Design review of the part built by this model. Coordinates are the model's own, in mm. A direction names the side the tool comes from. Give positions to 0.01 mm unless a question says otherwise; leave off trailing zeros. Write each loop counter-clockwise with the first axis right and the second up, starting at its lowest first coordinate (ties: lowest second). Pieces come first, ordered by that corner, then holes. Notation, with made-up numbers: (66.25, 55.25) -> (113.25, 55.25) arc R27 ccw to (113.25, 91.25) -> close; hole circle Ø6 at (-7.75, -39.75). An arc over 180 degrees is marked (long way). Put each result on its own line as item: value. Start each with the question number.
Autodesk Inventor part; units mm, degrees
ref_plane "YZ Plane" through (0, 0, 0) normal (1, 0, 0) x (0, 1, 0)
ref_plane "XZ Plane" through (0, 0, 0) normal (0, 1, 0) x (-1, 0, 0)
ref_plane "XY Plane" through (0, 0, 0) normal (0, 0, 1) x (1, 0, 0)
sketch "Sketch1" plane through (0, 0, 0) normal (0, 1, 0) x (-1, 0, 0)
  line L0 (11.1125, 9.525) -> (-11.1125, 9.525)
  line L1 (-11.1125, 9.525) -> (-11.1125, -9.525)
  line L2 (-11.1125, -9.525) -> (11.1125, -9.525)
  line L3 (11.1125, -9.525) -> (11.1125, 9.525)
  line L4 (11.1125, 9.525) -> (-11.1125, -9.525) construction
  line L5 (-11.1125, 9.525) -> (11.1125, -9.525) construction
  point P0 (0, 0)
  dimension "d0" = 22.225
  dimension "d1" = 19.05
extrude "Plate1" add sketch "Sketch1" along normal blind 1.524
sketch "Sketch2" plane through (-11.1125, 0, -8.001) normal (0, 0, -1) x (-1, 0, 0)
  line L0 (-22.225, 0) -> (0, 0)
  line L1 (0, 0) -> (0, 15.875)
  line L2 (0, 15.875) -> (-22.225, 15.875)
  line L3 (-22.225, 15.875) -> (-22.225, 0)
edge flange "Flange1" height 15.875 angle 90 thickness 1.524 bend radius 1.524 thickness toward (0, 0, -1) relief tear relief width 1.524 relief depth 0.762 edges at (0, 1.524, -9.525) wall of the first edge with corners at (11.1125, 0, -8.001) (-11.1125, 0, -8.001) (-11.1125, 15.875, -8.001) (11.1125, 15.875, -8.001)
bend "Bend1"
corner "Corner1"
sketch "Sketch3" plane through (0, 1.524, 0) normal (0, 1, 0) x (1, 0, 0)
  line L0 (11.1125, 6.477) -> (-11.1125, 6.477)
  line L1 (-11.1125, -9.525) -> (-11.1125, 6.477)
  line L2 (11.1125, -9.525) -> (-11.1125, -9.525)
  line L3 (11.1125, 6.477) -> (11.1125, -9.525)
  line L4 (-11.1125, -1.524) -> (11.1125, -1.524) construction
  line L5 (0, 6.477) -> (0, -9.525) construction
  circle A0 centre (0, -1.524) radius 2.2479
  line L6 (-5.1562, -1.524) -> (5.1562, -1.524) construction
  line L7 (-5.1562, 0.7239) -> (5.1562, 0.7239)
  line L8 (5.1562, -3.7719) -> (-5.1562, -3.7719)
  arc A1 (-5.1562, 0.7239) -> (-5.1562, -3.7719) centre (-5.1562, -1.524) ccw
  arc A2 (5.1562, -3.7719) -> (5.1562, 0.7239) centre (5.1562, -1.524) ccw
  point P0 (0, 0)
  dimension "d13" = 16.002
  dimension "d14" = 22.225
  dimension "d24" = 4.4958
  dimension "d25" = 3.7084
sketch "Sketch4" plane through (-11.1125, 15.875, -8.001) normal (0, 0, 1) x (1, 0, 0)
  line L0 (0, -12.827) -> (22.225, -12.827)
  line L1 (22.225, 0) -> (22.225, -12.827)
  line L2 (22.225, 0) -> (0, 0)
  line L3 (0, 0) -> (0, -12.827)
  line L4 (0, -6.4135) -> (22.225, -6.4135) construction
  line L5 (22.225, 0) -> (22.225, -12.827) construction
  line L6 (11.1125, -12.827) -> (11.1125, 0) construction
  line L7 (22.225, 0) -> (0, 0) construction
  point P0 (11.1125, -15.875)
  point P1 (11.1125, -6.4135)
  dimension "d15" = 22.225
  dimension "d16" = 12.827
hole "Hole1" at (0, 9.4615, -8.001) direction (0, 0, -1) diameter 4.4958 depth 1.524 tip angle 118
extrude "Cut1" cut sketch "Sketch3" against normal blind 1.524 contours A0 | A0 L7 A2 L8 | A0 L8 A1 L7
sketch "Sketch7" plane through (11.1125, 15.875, -9.525) normal (0, 0, -1) x (-1, 0, 0)
  line L0 (0, 0) -> (22.225, 0)
  line L1 (22.225, -15.875) -> (0, -15.875)
  line L2 (0, -12.827) -> (22.225, -12.827)
  point P0 (11.1125, -15.875)
  dimension "d28" = 15.875
  dimension "d29" = 12.827
  dimension "d30" = 22.225
sketch "Sketch8" plane through (0, 0, 0) normal (0, -1, 0) x (1, 0, 0)
  arc A0 (-5.1562, 3.7719) -> (-5.1562, -0.7239) centre (-5.1562, 1.524) ccw
  line L0 (-5.1562, 3.7719) -> (5.1562, 3.7719)
  arc A1 (5.1562, -0.7239) -> (5.1562, 3.7719) centre (5.1562, 1.524) ccw
  line L1 (5.1562, -0.7239) -> (-5.1562, -0.7239)
  line L2 (-11.1125, -6.477) -> (11.1125, -6.477)
  line L3 (11.1125, 9.525) -> (11.1125, -6.477)
  line L4 (-11.1125, 9.525) -> (11.1125, 9.525)
  line L5 (-11.1125, -6.477) -> (-11.1125, 9.525)
  line L6 (11.1125, -9.525) -> (-11.1125, -9.525)
  line L7 (11.1125, -6.477) -> (11.1125, -9.525)
  line L8 (-11.1125, -6.477) -> (11.1125, -6.477)
  line L9 (-11.1125, -9.525) -> (-11.1125, -6.477)
  point P0 (0, 0)
  dimension "d31" = 19.05
  dimension "d32" = 16.002
sketch "Sketch9" plane through (0, 1.524, 0) normal (0, 1, 0) x (1, 0, 0)
  arc A0 (5.1562, -3.7719) -> (5.1562, 0.7239) centre (5.1562, -1.524) ccw
  arc A1 (-5.1562, 0.7239) -> (-5.1562, -3.7719) centre (-5.1562, -1.524) ccw
  line L0 (5.1562, -3.7719) -> (-5.1562, -3.7719)
  line L1 (-5.1562, 0.7239) -> (5.1562, 0.7239)
  circle A2 centre (0, -1.524) radius 2.2479
  point P0 (0, 0)
  dimension "d34" = 5.1562
sketch "Sketch10" plane through (-11.1125, 15.875, -9.525) normal (0, 1, 0) x (1, 0, 0)
  line L0 (22.225, -19.05) -> (0, -19.05)
  line L1 (22.225, 0) -> (0, 0)
  line L2 (0, -1.524) -> (0, 0)
  line L3 (0, -1.524) -> (0, -3.048)
  line L4 (0, -19.05) -> (0, -3.048)
  line L5 (0, 0) -> (7.1374, 0)
  line L6 (7.1374, 0) -> (7.1374, -19.05)
  line L7 (7.1374, -19.05) -> (0, -19.05)
  line L8 (0, -19.05) -> (0, 0)
  line L9 (22.225, 0) -> (15.0876, 0)
  line L10 (15.0876, 0) -> (15.0876, -19.05)
  line L11 (15.0876, -19.05) -> (22.225, -19.05)
  line L12 (22.225, -19.05) -> (22.225, 0)
  point P0 (11.1125, -9.525)
  dimension "d35" = 7.1374
  dimension "d36" = 7.1374
equation "\"d22\" = Thickness"
equation "\"d26\" = Thickness"
equation "\"d36\" = d35"
equation "\"d3\" = BendReliefWidth"
equation "\"d4\" = BendReliefDepth"
equation "\"d5\" = MinimumRemnant"
equation "\"d6\" = BendRadius"
equation "\"d9\" = BendRadius"
equation "\"d10\" = CornerReliefSize"
equation "\"d11\" = GapSize"
equation "\"d12\" = JacobiRadiusSize"
equation "\"BendRadius\" = Thickness"
equation "\"BendReliefWidth\" = Thickness"
equation "\"BendReliefDepth\" = 0.5 * Thickness"
equation "\"CornerReliefSize\" = 4 * Thickness"
equation "\"MinimumRemnant\" = 2 * Thickness"
equation "\"TransitionRadius\" = BendRadius"
equation "\"JacobiRadiusSize\" = BendRadius"
equation "\"GapSize\" = Thickness"
equation "\"d2\" = BendRadius"
properties part number "Bracket (15275A53)" material "Steel"
Q1. Take a section at A-A on x = 0. Give the boundary of the cut face in (y, z) (3 decimals).
Q2. To check wall thickness, follow probe 1 along Z at (x, y) = (5, 13) (3 decimals); probe 2 along Y at (x, z) = (9.75, 3.5); probe 3 along Z at (x, y) = (-1.25, 0.5) (3 decimals). State the ranges of each line that lie inside material, in increasing order. Write a range as from..to.
Q3. Take a section at D-D on z = 0.75. Give the boundary of the cut face in (x, y), then the cut area to 3 significant figures.
Q4. Take a section at B-B on y = 8.75. Give the boundary of the cut face in (x, z) (1 decimal), then the cut area to 3 significant figures.
Q5. For pin 1 (6.5 mm diameter, centred on x = -0.5, y = 6.5, fed in from +Z); pin 2 (0.8 mm diameter, centred on x = 0.5, y = 0.5, fed in from -Z); pin 3 (2 mm diameter, centred on x = 3, z = -2.5, fed in from +Y), all flat-tipped, find the tip position at first contact; note any pin that passes through.
Q6. Take a section at C-C on x = 6.75. Give the boundary of the cut face in (y, z) (3 decimals).
Q7. Machinability: for faces 4 (the face through (0, 1, 9.525)), 5 (the face through (0, 1.524, -2)), 6 (the face through (-7.404, 0.773, 1.475)), which of the approach directions +Z, -Z, +X, -X, +Y, -Y give a long, thin tool a straight path to every point of the face, cutting with its end or side? Answer none if there is none.
Q8. Mouldability with a two-part tool opening along Z and no side actions: class faces 1 (the face through (0, 1, -0.724)), 2 (the face through (0, 15.875, -9)), 3 (the face through (-0.156, 1.982, -7.566)) as +Z half, -Z half, draft (parallel to the pull), parting line (faces both ways), or undercut.
Result:
1. outline: (0, -6.477) arc R3.048 ccw to (3.048, -9.525) -> (7.214, -9.525) -> (7.214, -8.001) -> (3.048, -8.001) arc R1.524 cw to (1.524, -6.477) -> (1.524, -0.724) -> (0, -0.724) -> close; (0, 3.772) -> (1.524, 3.772) -> (1.524, 9.525) -> (0, 9.525) -> close; (11.709, -9.525) -> (15.875, -9.525) -> (15.875, -8.001) -> (11.709, -8.001) -> close
2. probe 1: z = -9.525..-8.001
2. probe 2: y = 0..1.52
2. probe 3: z = -8.15..-0.724, 3.772..9.525
3. outline: (-11.11, 0) -> (-7.27, 0) -> (-7.27, 1.52) -> (-11.11, 1.52) -> close; (7.27, 0) -> (11.11, 0) -> (11.11, 1.52) -> (7.27, 1.52) -> close
3. area: 11.7 mm^2
4. outline: (-11.1, -9.5) -> (-2.1, -9.5) -> (-2.1, -8) -> (-11.1, -8) -> close; (2.1, -9.5) -> (11.1, -9.5) -> (11.1, -8) -> (2.1, -8) -> close
4. area: 27.4 mm^2
5. pin 1: stops at z = -8
5. pin 2: stops at z = -8.64
5. pin 3: stops at y = 1.52
6. outline: (0, -6.477) arc R3.048 ccw to (3.048, -9.525) -> (15.875, -9.525) -> (15.875, -8.001) -> (3.048, -8.001) arc R1.524 cw to (1.524, -6.477) -> (1.524, -0.061) -> (0, -0.061) -> close; (0, 3.109) -> (1.524, 3.109) -> (1.524, 9.525) -> (0, 9.525) -> close
7. face 4: +Z, +X, -X, +Y, -Y
7. face 5: +Z, +X, -X, +Y
7. face 6: +Y, -Y
8. face 1: undercut
8. face 2: draft
8. face 3: +Z half
